Input: part model. Units: mm. Frame: model coordinates. A direction names the side the tool comes from. Give positions to 0.01 mm unless a question says otherwise; leave off trailing zeros. Write each loop counter-clockwise with the first axis right and the second up, starting at its lowest first coordinate (ties: lowest second). Pieces come first, ordered by that corner, then holes. Notation, with made-up numbers: (79, -20.75) - (110, -20.75) arc R28 cw to (110, 13.25) - close; hole circle Ø1 at (62, 62). An arc over 180 degrees is marked (long way). Answer as a JSON object with one key per item and string values. Group by question number.
from build123d import *

# Parameters (mm, degrees)
SKETCH1_W                                           = 190
SKETCH1_H                                           = 220
SKETCH1_W_2                                         = 130
SKETCH1_H_2                                         = 160
BOSS_EXTRUDE1_DEPTH                                 = 6.35
CSK_FOR_M6_COUNTERSUNK_FLAT_HEAD_SCREW1_D           = 6.6
CSK_FOR_M6_COUNTERSUNK_FLAT_HEAD_SCREW1_DEPTH       = 45
CSK_FOR_M6_COUNTERSUNK_FLAT_HEAD_SCREW1_CSINK_D     = 12.5984
CSK_FOR_M6_COUNTERSUNK_FLAT_HEAD_SCREW1_CSINK_ANGLE = 90
CSK_FOR_M6_COUNTERSUNK_FLAT_HEAD_SCREW1_TIP         = 1.982840043


with BuildPart() as part:
    # Sketch1 → Boss-Extrude1 (new body)
    with BuildSketch(Plane.XY):
        Rectangle(SKETCH1_W, SKETCH1_H)
        Rectangle(SKETCH1_W_2, SKETCH1_H_2, mode=Mode.SUBTRACT)
    extrude(amount=BOSS_EXTRUDE1_DEPTH)

    # CSK for M6 Countersunk Flat Head Screw1
    with Locations(Plane.XY.offset(6.35)):
        with Locations((-85, -70), (-85, 100), (85, 100), (85, -70)):
            CounterSinkHole(CSK_FOR_M6_COUNTERSUNK_FLAT_HEAD_SCREW1_D / 2, CSK_FOR_M6_COUNTERSUNK_FLAT_HEAD_SCREW1_CSINK_D / 2, depth=CSK_FOR_M6_COUNTERSUNK_FLAT_HEAD_SCREW1_DEPTH, counter_sink_angle=CSK_FOR_M6_COUNTERSUNK_FLAT_HEAD_SCREW1_CSINK_ANGLE)
            with Locations((0, 0, -(CSK_FOR_M6_COUNTERSUNK_FLAT_HEAD_SCREW1_DEPTH + CSK_FOR_M6_COUNTERSUNK_FLAT_HEAD_SCREW1_TIP / 2))):  # 118° drill point
                Cone(0, CSK_FOR_M6_COUNTERSUNK_FLAT_HEAD_SCREW1_D / 2, CSK_FOR_M6_COUNTERSUNK_FLAT_HEAD_SCREW1_TIP, mode=Mode.SUBTRACT)


solid = part.part
1) Mould query, pull axis Y, two halves, no side actions, for faces 1 (the face through (87.43, -67.77, 1.65)), 2 (the face through (70, 9, 6.35)), 3 (the face through (-1, 110, 3)). Classes: +Y half, -Y half, draft (parallel to the pull), parting line (faces both ways), or undercut.
2) Cut plane B-B on x = 85. Return the cut outline in (y, z), and give its area (3 significant figures).
3) Cut plane A-A on y = 31.5. Return the cut outline in (x, z).
4) Reachability of faces 4 (the face through (88.442, 100.151, 3.496)), 5 (the face through (-1, 80, 3)) from +Z, -Z, +X, -X, +Y, -Y: full face, straight path, thin tool, end or side. Return the list, or none.
5) Cut plane D-D on x = -36.5. Return the cut outline in (y, z), and give its area (3 significant figures).
6) Cut plane C-C on y = 100. Return the cut outline in (x, z).
7) Line query: line 1 along Y through (x, z) = (85, 0.7); line 2 along X through (y, z) = (-70, 1.3); line 3 along X through (y, z) = (100, 2). Output: solid intervals per line, ascending. Write a range as from..to.
Filled in:
{
 "1": {"face 1": "undercut", "face 2": "draft", "face 3": "+Y half"},
 "2": {"outline": "(-110, 0) - (-73.3, 0) - (-73.3, 3.35) - (-76.3, 6.35) - (-110, 6.35) - close; (-66.7, 0) - (96.7, 0) - (96.7, 3.35) - (93.7, 6.35) - (-63.7, 6.35) - (-66.7, 3.35) - close; (103.3, 0) - (110, 0) - (110, 6.35) - (106.3, 6.35) - (103.3, 3.35) - close", "area": "1,300 mm²"},
 "3": {"outline": "(-95, 0) - (-65, 0) - (-65, 6.35) - (-95, 6.35) - close; (65, 0) - (95, 0) - (95, 6.35) - (65, 6.35) - close"},
 "4": {"face 4": "+Z", "face 5": "+Z, -Z"},
 "5": {"outline": "(-110, 0) - (-80, 0) - (-80, 6.35) - (-110, 6.35) - close; (80, 0) - (110, 0) - (110, 6.35) - (80, 6.35) - close", "area": "381 mm²"},
 "6": {"outline": "(-95, 0) - (-88.3, 0) - (-88.3, 3.35) - (-91.3, 6.35) - (-95, 6.35) - close; (-81.7, 0) - (81.7, 0) - (81.7, 3.35) - (78.7, 6.35) - (-78.7, 6.35) - (-81.7, 3.35) - close; (88.3, 0) - (95, 0) - (95, 6.35) - (91.3, 6.35) - (88.3, 3.35) - close"},
 "7": {"line 1": "y = -110..-73.3, -66.7..96.7, 103.3..110", "line 2": "x = -95..-88.3, -81.7..-65, 65..81.7, 88.3..95", "line 3": "x = -95..-88.3, -81.7..81.7, 88.3..95"}
}
